Source: CAD feature listing. Evaluate the final solid. Frame: model axes, mm. A direction names the side the tool comes from. Coordinates: 2 decimals unless noted, no trailing zeros. Write each loop counter-clockwise with the first axis right and the second up, starting at its lowest first coordinate (ties: lowest second). Pieces come first, ordered by that corner, then holes. Notation, with made-up numbers: (21, 47) - (78, 47) arc R17 cw to (78, 53) - close; hole circle Ø5 at (-33, 78.25). An arc over 180 degrees is marked (long way). One line per item, written item: value.
Autodesk Inventor part; units mm, degrees
ref_plane "YZ Plane" through (0, 0, 0) normal (1, 0, 0) x (0, 1, 0)
ref_plane "XZ Plane" through (0, 0, 0) normal (0, 1, 0) x (-1, 0, 0)
ref_plane "XY Plane" through (0, 0, 0) normal (0, 0, 1) x (1, 0, 0)
sketch "Sketch1" plane through (0, 0, 0) normal (0, 0, 1) x (1, 0, 0)
  line L0 (-16, 12.5) -> (-13, 12.5)
  line L1 (-13, 12.5) -> (-13, -9.5)
  line L2 (-13, -9.5) -> (13, -9.5)
  line L3 (13, -9.5) -> (13, 12.9)
  line L4 (13, 12.9) -> (16, 12.9)
  line L5 (16, 12.9) -> (16, -12.5)
  line L6 (16, -12.5) -> (-16, -12.5)
  line L7 (-16, -12.5) -> (-16, 12.5)
  point P0 (0, 0)
  dimension "d0" = 3
  dimension "d2" = 3
  dimension "d3" = 25
  dimension "d4" = 32
  dimension "d5" = 16
  dimension "d7" = 12.5
  dimension "d8" = 3
extrude "Extrusion1" add sketch "Sketch1" against normal blind 481.1268
sketch "Sketch4" plane through (-16, -12.5, 0) normal (0, -1, 0) x (1, 0, 0)
  line L0 (32, 0) -> (0, 0)
  line L1 (32, -481.1268) -> (0, -481.1268)
  line L2 (32, 0) -> (32, -481.1268)
  circle A0 centre (16, -12.5) radius 3.175
  circle A1 centre (16, -468.6268) radius 3.175
  point P0 (16, 0)
  dimension "d21" = 6.35
  dimension "d22" = 6.35
  dimension "d23" = 12.5
  dimension "d24" = 12.5
  dimension "d25" = 16
hole "Hole1" at (0, -12.5, -12.5) at (0, -12.5, -468.6268) direction (0, 1, 0) diameter 6.35 depth 3 tip angle 118
equation "\"d2\" = d0"
equation "\"d8\" = d0"
equation "\"d24\" = d23"
properties part number "19in c-channel"
1) Material intervals for line 1 (Z direction, x = 0, y = -10.7) (3 decimals); line 2 (X direction, y = -0.75, z = -223); line 3 (X direction, y = -11.9, z = -12.5) (3 decimals), sorted ascending.
Values found:
line 1: -481.127 to -471.802, -465.452 to -15.675, -9.325 to 0
line 2: -16 to -13, 13 to 16
line 3: -16 to -3.175, 3.175 to 16
2) Section query B-B on z = -306.5. Output: boundary loops of the cut face in (x, y), then the cut area to 3 significant figures.
Values found:
outline: (-16, -12.5) - (16, -12.5) - (16, 12.9) - (13, 12.9) - (13, -9.5) - (-13, -9.5) - (-13, 12.5) - (-16, 12.5) - close
area: 229 mm2
3) Section query A-A on y = 4.5. Output: boundary loops of the cut face in (x, z), then the cut area to 3 significant figures.
Values found:
outline: (-16, -481.13) - (-13, -481.13) - (-13, 0) - (-16, 0) - close; (13, -481.13) - (16, -481.13) - (16, 0) - (13, 0) - close
area: 2,890 mm2
4) Draft query along X for faces 1 (the flat face through (-1, -10, 0)), 2 (the flat face through (16, 0, -237)), 3 (the flat face through (-13, 2, -237)). Return one class per face: released by +X, released by -X, zero draft, split by the parting line, or undercut.
Values found:
face 1: zero draft
face 2: released by +X
face 3: undercut
5) Contact query for flat-ended pins moving along their axis: P1, Ø8, axis at x = 5, z = -307.5, coming from the +Y side; P2, Ø8, axis at x = -8, y = 7, coming from the +Z side; P3, Ø0.9, axis at x = -14.5, z = -335.5, coming from the +Y side. Output: stop coordinate, or through.
Values found:
P1: y = -9.5
P2: through
P3: y = 12.5
6) Reachability of faces 4 (the flat face through (-16, 0, -237)), 5 (the flat face through (0, -9.5, -237)) from +Z, -Z, +X, -X, +Y, -Y: full face, straight path, thin tool, end or side. Return the list, or none.
Values found:
face 4: +Z, -Z, -X, +Y, -Y
face 5: +Z, -Z, +Y
